Model file for the job. Use its own axes, mm. Face numbers are marked on the shaded views. A direction names the side the tool comes from. Coordinates: 2 decimals unless noted, no trailing zeros. Loops run counter-clockwise (first coordinate to the right, second up) from the corner with the lowest first, then second, coordinate; pieces in that order, holes last.
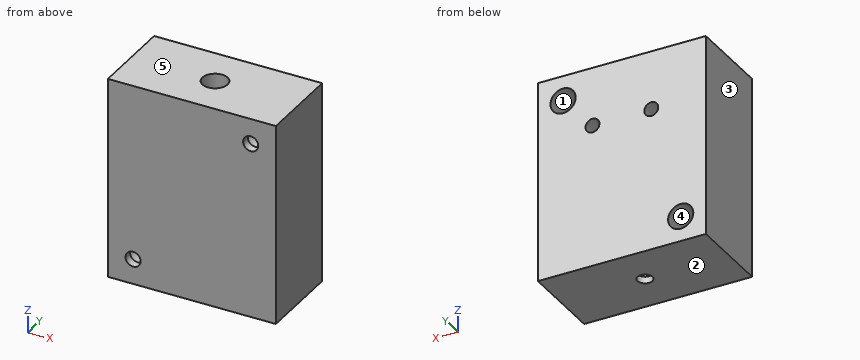
from build123d import *

# Parameters (mm, degrees)
SKIZZE1_W                                           = 100
SKIZZE1_H                                           = 50
AUFSATZ_LINEAR_AUSTRAGEN1_DEPTH                     = 120
STIRNSENKUNG_F_R_M8_SENKSCHRAUBE_KOPF_B_D           = 9
STIRNSENKUNG_F_R_M8_SENKSCHRAUBE_KOPF_B_CBORE_D     = 15
STIRNSENKUNG_F_R_M8_SENKSCHRAUBE_KOPF_B_CBORE_DEPTH = 45
STIRNSENKUNG_F_R_M8_SENKSCHRAUBE_KO_2_D             = 9
STIRNSENKUNG_F_R_M8_SENKSCHRAUBE_KO_2_CBORE_D       = 15
STIRNSENKUNG_F_R_M8_SENKSCHRAUBE_KO_2_CBORE_DEPTH   = 116
KERNLOCH_F_R_M8_HELICOIL1_D                         = 8.3
KERNLOCH_F_R_M8_HELICOIL1_DEPTH                     = 20
KERNLOCH_F_R_M8_HELICOIL1_TIP                       = 2.493571569


with BuildPart() as part:
    # Skizze1 → Aufsatz-Linear austragen1 (new body)
    with BuildSketch(Plane.XY):
        Rectangle(SKIZZE1_W, SKIZZE1_H)
    extrude(amount=AUFSATZ_LINEAR_AUSTRAGEN1_DEPTH)

    # Stirnsenkung f_r M8 Senkschraube _Kopf B (through all)
    with Locations(Plane(origin=(0, 25, 0), x_dir=(1, 0, 0), z_dir=(0, 1, 0))):
        with Locations((35, -105), (-35, -15)):
            CounterBoreHole(STIRNSENKUNG_F_R_M8_SENKSCHRAUBE_KOPF_B_D / 2, STIRNSENKUNG_F_R_M8_SENKSCHRAUBE_KOPF_B_CBORE_D / 2, STIRNSENKUNG_F_R_M8_SENKSCHRAUBE_KOPF_B_CBORE_DEPTH)

    # Stirnsenkung f_r M8 Senkschraube _Ko 2 (through all)
    with Locations(Plane.XY.offset(120)):
        with Locations((0, 0)):
            CounterBoreHole(STIRNSENKUNG_F_R_M8_SENKSCHRAUBE_KO_2_D / 2, STIRNSENKUNG_F_R_M8_SENKSCHRAUBE_KO_2_CBORE_D / 2, STIRNSENKUNG_F_R_M8_SENKSCHRAUBE_KO_2_CBORE_DEPTH)

    # Kernloch für M8 Helicoil1
    with Locations(Plane(origin=(0, 25, 0), x_dir=(1, 0, 0), z_dir=(0, 1, 0))):
        with Locations((-17.5, -85), (17.5, -85)):
            Hole(KERNLOCH_F_R_M8_HELICOIL1_D / 2, depth=KERNLOCH_F_R_M8_HELICOIL1_DEPTH)
            with Locations((0, 0, -(KERNLOCH_F_R_M8_HELICOIL1_DEPTH + KERNLOCH_F_R_M8_HELICOIL1_TIP / 2))):  # 118° drill point
                Cone(0, KERNLOCH_F_R_M8_HELICOIL1_D / 2, KERNLOCH_F_R_M8_HELICOIL1_TIP, mode=Mode.SUBTRACT)


solid = part.part
Q1. Flat gauge pins, fed straight in: P1, Ø13.5, axis at x = -35, z = 15, coming from the +Y side; P2, Ø12, axis at x = 0, y = 0, coming from the +Z side. Where does each tip first touch, or does it go through?
Answers:
P1: stops at y = -20
P2: stops at z = 4
Q2. Mould opens along X. For the marked faces 3, 4 and 5 say: +X half, -X half, draft (parallel to the pull), parting line (faces both ways), or undercut.
Answers:
face 3: -X half
face 4: undercut
face 5: draft
Q3. Which spindle directions (+Z, -Z, +X, -X, +Y, -Y) get a long thin tool onto all of the face, cutting with end or side? Do the marked faces 1 and 2. Say none if no direction does.
Answers:
face 1: +Y
face 2: -Z, +X, -X, +Y, -Y
Q4. Slice it at A-A (x = 0). List the corners of the cut face in (y, z).
Answers:
outline: (-25, 0) - (-4.5, 0) - (-4.5, 4) - (-7.5, 4) - (-7.5, 120) - (-25, 120) - close; (4.5, 0) - (25, 0) - (25, 120) - (7.5, 120) - (7.5, 4) - (4.5, 4) - close
Q5. Slice it at B-B (z = 105). List the corners of the cut face in (x, y).
Answers:
outline: (-50, -25) - (30.5, -25) - (30.5, -20) - (27.5, -20) - (27.5, 25) - (-50, 25) - close; (39.5, -25) - (50, -25) - (50, 25) - (42.5, 25) - (42.5, -20) - (39.5, -20) - close; hole circle Ø15 at (0, 0)
Q6. Slice it at D-D (z = 21). List the corners of the cut face in (x, y), and give its area (3 significant figures).
Answers:
outline: (-50, -25) - (50, -25) - (50, 25) - (-30.5, 25) - (-30.5, -20) - (-39.5, -20) - (-39.5, 25) - (-50, 25) - close; hole circle Ø15 at (0, 0)
area: 4,420 mm2
Q7. Drill centre lines: line 1 (X direction, y = 11.5, z = 85); line 2 (X direction, y = -2, z = 105); line 3 (Y direction, x = 0, z = 50). Where is each one in solid material? Low to high.
Answers:
line 1: x = -50 to -21.65, -13.35 to 13.35, 21.65 to 50
line 2: x = -50 to -7.23, 7.23 to 27.5, 42.5 to 50
line 3: y = -25 to -7.5, 7.5 to 25
Q8. Slice it at C-C (y = 13). List the corners of the cut face in (x, z).
Answers:
outline: (-50, 0) - (50, 0) - (50, 120) - (-50, 120) - close; hole circle Ø15 at (-35, 15); hole circle Ø8.3 at (-17.5, 85); hole circle Ø8.3 at (17.5, 85); hole circle Ø15 at (35, 105)
